Geometry: final body of the model. Coordinates: model frame, mm. Face numbers are marked on the shaded views. Give positions to 0.01 mm unless a question says otherwise; leave off trailing zeros. Write each loop counter-clockwise with the first axis right and the second up, starting at its lowest first coordinate (ties: lowest second). Pieces come first, ordered by that corner, then holes.
Q1. Cut plane B-B on y = -44. Return the cut outline in (x, z).
Q2. Cut plane D-D on z = 733. Return the cut outline in (x, y), plus the area to 3 significant figures.
Q3. Line query: L1, parallel to X at y = 35.5, z = 551; L2, parallel to Y at x = -16.9, z = -2; L3, parallel to Z at x = -62, y = 97. Output: solid intervals per line, ascending.
Q4. Pin query (flat end, axial travel): pin 1 (2 mm diameter, centred on x = -72, y = -43.5, fed in from -Z); pin 2 (1.2 mm diameter, centred on x = 37, z = 394, fed in from +Y); pin 3 (1 mm diameter, centred on x = -9.5, z = 74.5, fed in from -Y). Return the tip coordinate at first contact, or that it passes through.
Q5. Cut plane C-C on x = -62. Return the cut outline in (y, z), plus the area to 3 significant figures.
Q6. Draft query along Z for the marked faces 1 and 2. Return one class per face: pulls with the +Z half, pulls with the -Z half, needs draft (parallel to the pull), parting line crosses it, or undercut.
Q7. Cut plane A-A on z = 365.5. Return the cut outline in (x, y), plus the area to 3 significant figures.
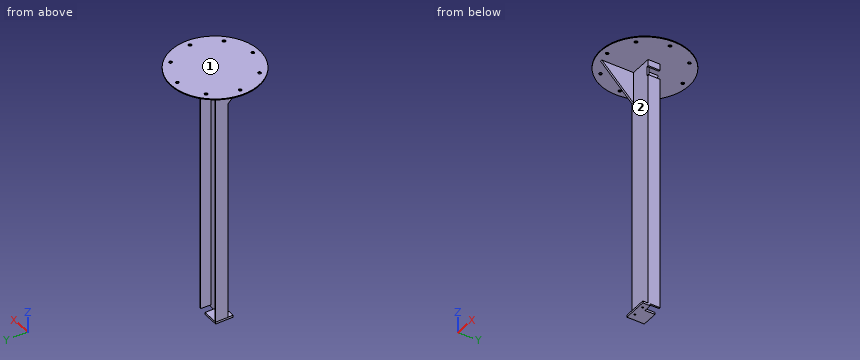
```python
from build123d import *

# Parameters (mm, degrees)
BOSS_EXTRUDE1_DEPTH = 800
SKETCH4_W           = 50
SKETCH4_H           = 38.1
CUT_EXTRUDE2_DEPTH  = 5.6
SKETCH5_R           = 4
BOSS_EXTRUDE2_DEPTH = 30
SKETCH6_W           = 20
SKETCH6_H           = 38.1
BOSS_EXTRUDE3_DEPTH = 5
SKETCH7_W           = 76
SKETCH7_H           = 55.1
BOSS_EXTRUDE4_DEPTH = 6.35
SKETCH8_R           = 139.7
BOSS_EXTRUDE5_DEPTH = 3
SKETCH9_W           = 25
SKETCH9_H           = 31.75
CUT_EXTRUDE3_DEPTH  = 6.35
SKETCH10_R          = 2.75
CUT_EXTRUDE4_DEPTH  = 6.35
CUT_EXTRUDE5_REACH  = 837.76
SKETCH11_R          = 5
CIRPATTERN1_COUNT   = 8
BOSS_EXTRUDE6_DEPTH = 6


with BuildPart() as part:
    # Sketch1 → Boss-Extrude1 (new body)
    with BuildSketch(Plane.XY):
        Polygon((38.1, 0), (-38.1, 0), (-38.1, 38.1), (-34.1, 38.1), (-32.5, 6.35), (32.5, 6.35), (34.1, 38.1), (38.1, 38.1), align=None)
    extrude(amount=BOSS_EXTRUDE1_DEPTH)

    # Sketch4 → Cut-Extrude2 (cut)
    with BuildSketch(Plane(origin=(38.1, 0, 0), x_dir=(0, 0, -1), z_dir=(1, 0, 0))):
        with Locations((-775, 19.05)):
            Rectangle(SKETCH4_W, SKETCH4_H)
    extrude(amount=-CUT_EXTRUDE2_DEPTH, mode=Mode.SUBTRACT)

    # Sketch5 → Boss-Extrude2 (add)
    with BuildSketch(Plane(origin=(0, 6.35, 0), x_dir=(1, 0, 0), z_dir=(0, 1, 0))):
        with Locations(Location((26.1, -765, 0), (0, 0, 90))):
            Circle(SKETCH5_R)
    extrude(amount=BOSS_EXTRUDE2_DEPTH)

    # Sketch6 → Boss-Extrude3 (add)
    with BuildSketch(Plane(origin=(32.5, 0, 0), x_dir=(0, 0, -1), z_dir=(1, 0, 0))):
        with Locations((-790, 19.05)):
            Rectangle(SKETCH6_W, SKETCH6_H)
    extrude(amount=BOSS_EXTRUDE3_DEPTH)

    # Sketch7 → Boss-Extrude4 (add)
    with BuildSketch(Plane(origin=(0, 0, 0), x_dir=(-1, 0, 0), z_dir=(0, 0, -1))):
        with Locations((-0.1, 10.55)):
            Rectangle(SKETCH7_W, SKETCH7_H)
    extrude(amount=BOSS_EXTRUDE4_DEPTH)

    # Sketch8 → Boss-Extrude5 (add)
    with BuildSketch(Plane.XY.offset(800)):
        with Locations((0, 15)):
            Circle(SKETCH8_R)
    extrude(amount=BOSS_EXTRUDE5_DEPTH)

    # Sketch9 → Cut-Extrude3 (cut)
    with BuildSketch(Plane(origin=(0, 0, -6.35), x_dir=(-1, 0, 0), z_dir=(0, 0, -1))):
        with Locations((-25.6, 22.225)):
            Rectangle(SKETCH9_W, SKETCH9_H)
    extrude(amount=-CUT_EXTRUDE3_DEPTH, mode=Mode.SUBTRACT)

    # Sketch10 → Cut-Extrude4 (cut)
    with BuildSketch(Plane(origin=(0, 0, -6.35), x_dir=(-1, 0, 0), z_dir=(0, 0, -1))):
        with Locations((-21.1, -6)):
            Circle(SKETCH10_R)
        with Locations((16.9, -6)):
            Circle(SKETCH10_R)
    extrude(amount=-CUT_EXTRUDE4_DEPTH, mode=Mode.SUBTRACT)

    # Sketch11 → Cut-Extrude5 (cut, up to next)
    with BuildSketch(Plane.XY.offset(803), mode=Mode.PRIVATE) as cut_extrude5_sk1:
        with Locations((0, 134.7)):
            Circle(SKETCH11_R)
    cut_extrude5_tool1 = extrude(cut_extrude5_sk1.sketch, amount=-CUT_EXTRUDE5_REACH, mode=Mode.PRIVATE) & part.part
    cut_extrude5 = cut_extrude5_tool1.solids().sort_by_distance((0, 134.7, 803))[0]
    add(cut_extrude5, mode=Mode.SUBTRACT)

    # CirPattern1: Cut-Extrude5 ×8 about axis
    cirpattern1_axis = Axis((0, 15, 0), (0, 0, 1))
    for i in range(1, CIRPATTERN1_COUNT):
        add(cut_extrude5.rotate(cirpattern1_axis, i * 360 / CIRPATTERN1_COUNT), mode=Mode.SUBTRACT)

    # Sketch12 → Boss-Extrude6 (add)
    with BuildSketch(Plane.ZY.offset(38.1)):
        Polygon((700, 0), (800, -100), (800, 0), align=None)
    extrude(amount=-BOSS_EXTRUDE6_DEPTH)


solid = part.part
```
Data:
1. outline: (-126.63, 800) - (-38.1, 800) - (-38.1, 744) - (-32.1, 744) - (-32.1, 800) - (126.63, 800) - (126.63, 803) - (-126.63, 803) - close
2. outline: (-38.1, -33) - (-32.1, -33) - (-32.1, 0) - (38.1, 0) - (38.1, 38.1) - (34.1, 38.1) - (32.5, 6.35) - (-32.5, 6.35) - (-34.1, 38.1) - (-38.1, 38.1) - close
2. area: 987 mm2
3. L1: x = -38.1 to -33.97, 33.97 to 38.1
3. L2: y = -17 to -8.75, -3.25 to 38.1
3. L3: z = 800 to 803
4. pin 1: stops at z = 800
4. pin 2: stops at y = 38.1
4. pin 3: stops at y = 0
5. outline: (-110.19, 800) - (140.19, 800) - (140.19, 803) - (-110.19, 803) - close
5. area: 751 mm2
6. face 1: pulls with the +Z half
6. face 2: undercut
7. outline: (-38.1, 0) - (38.1, 0) - (38.1, 38.1) - (34.1, 38.1) - (32.5, 6.35) - (-32.5, 6.35) - (-34.1, 38.1) - (-38.1, 38.1) - close
7. area: 789 mm2
